The listing builds one solid part. Answer for the finished solid, in the listing's coordinates (mm). Give positions to 0.01 mm unless a question says otherwise; leave off trailing zeros. Write each loop counter-clockwise with the first axis right and the second up, starting at its lowest first coordinate (ties: lowest second). Pieces come first, ordered by that corner, then holes. Notation, with made-up numbers: (-0.75, 23.5) - (58.25, 23.5) arc R27 ccw to (58.25, 62.5) - close; hole circle Ø7 at (41, -28). An arc over 180 degrees is marked (long way). Write each question's results on one line, items separated by ' | '. Start each with the question number.
Q1. Section D-D (z = 1.5) is taken. Determine the outline of the cut face in (x, y), plus the area to 3 significant figures.
Q2. Section B-B (z = 4) is taken. Determine the outline of the cut face in (x, y), plus the area to 3 significant figures.
Q3. For a pull along Y with two mould halves and no side action, classify faces 1 (the face through (15, 0, 5)), 2 (the face through (23.88, 3.55, 4.56)), 3 (the face through (14.226, 4.21, 5.07)) as pulls with the +Y half, pulls with the -Y half, needs draft (parallel to the pull), parting line crosses it, or undercut.
Q4. Find the intervals of material crossed by probe 1 along X at (y, z) = (5.25, 5); probe 2 along Y at (x, z) = (15, 4.25); probe 3 along Z at (x, y) = (22.5, 3.25), in increasing order.
Q5. Section A-A (y = 3.5) is taken. Determine the outline of the cut face in (x, z).
Q6. Section C-C (x = 15) is taken. Determine the outline of the cut face in (y, z), plus the area to 3 significant figures.
Q7. Flat-ended cylindrical pins translate along their axes: pin 1 Ø1.5 at (x, y) = (5.5, 0.5) entering from -Z; pin 2 Ø2.5 at (x, z) = (22.5, 5) entering from +Y. Find the tip coordinate at first contact, or state that the pin passes through.
```python
from build123d import *

# Parameters (mm, degrees)
SKETCH1_W           = 30
SKETCH1_H           = 7
BOSS_EXTRUDE1_DEPTH = 10
SKETCH2_R           = 1.05
CUT_EXTRUDE1_DEPTH  = 10
SKETCH3_R           = 1.45
CUT_EXTRUDE2_DEPTH  = 8


with BuildPart() as part:
    # Sketch1 → Boss-Extrude1 (new body)
    with BuildSketch(Plane.XY):
        with Locations((15, 3.5)):
            Rectangle(SKETCH1_W, SKETCH1_H)
    extrude(amount=BOSS_EXTRUDE1_DEPTH)

    # Sketch2 → Cut-Extrude1 (cut)
    with BuildSketch(Plane.XY.offset(10)):
        with Locations((15, 3.5)):
            Circle(SKETCH2_R)
    extrude(amount=-CUT_EXTRUDE1_DEPTH, mode=Mode.SUBTRACT)

    # Sketch3 → Cut-Extrude2 (cut, through all)
    with BuildSketch(Plane(origin=(0, 7, 0), x_dir=(1, 0, 0), z_dir=(0, 1, 0))):
        with Locations((7.5, -5)):
            Circle(SKETCH3_R)
        with Locations((22.5, -5)):
            Circle(SKETCH3_R)
    extrude(amount=-CUT_EXTRUDE2_DEPTH, mode=Mode.SUBTRACT)


solid = part.part
```
Answers below:
1) outline: (0, 0) - (30, 0) - (30, 7) - (0, 7) - close; hole circle Ø2.1 at (15, 3.5) | area: 207 mm2
2) outline: (0, 0) - (6.45, 0) - (6.45, 7) - (0, 7) - close; (8.55, 0) - (21.45, 0) - (21.45, 7) - (8.55, 7) - close; (23.55, 0) - (30, 0) - (30, 7) - (23.55, 7) - close; hole circle Ø2.1 at (15, 3.5) | area: 177 mm2
3) face 1: pulls with the -Y half | face 2: needs draft | face 3: undercut
4) probe 1: x = 0 to 6.05, 8.95 to 21.05, 23.95 to 30 | probe 2: y = 0 to 2.45, 4.55 to 7 | probe 3: z = 0 to 3.55, 6.45 to 10
5) outline: (0, 0) - (13.95, 0) - (13.95, 10) - (0, 10) - close; (16.05, 0) - (30, 0) - (30, 10) - (16.05, 10) - close; hole circle Ø2.9 at (7.5, 5); hole circle Ø2.9 at (22.5, 5)
6) outline: (0, 0) - (2.45, 0) - (2.45, 10) - (0, 10) - close; (4.55, 0) - (7, 0) - (7, 10) - (4.55, 10) - close | area: 49.0 mm2
7) pin 1: stops at z = 0 | pin 2: passes through
